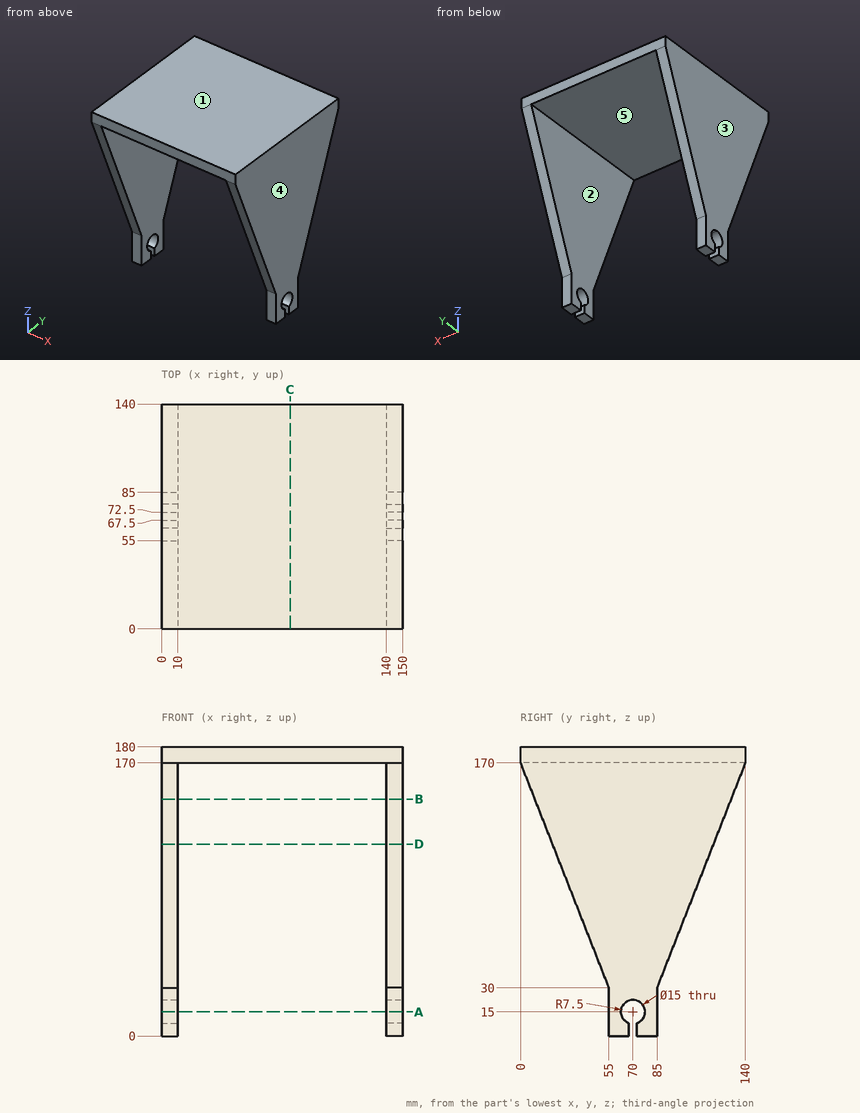
Source: three-view drawing plus pictorial views. Frame: mm from the lowest corner of the part. A direction names the side the tool comes from. Round coordinates to 2 decimals unless told otherwise and drop trailing zeros. Loops run counter-clockwise (first coordinate to the right, second up) from the corner with the lowest first, then second, coordinate; pieces in that order, holes last. Notation, with made-up numbers: (-28.5, 75.5) - (9.5, 75.5) arc R24 cw to (9.5, 87.5) - close; hole circle Ø7 at (63, 49.5). An arc over 180 degrees is marked (long way). Write each question's results on one line, items separated by ' | '. Start each with the question number.
1) Cut plane C-C on x = 80. Return loops of the section in (y, z).
2) Cut plane A-A on z = 15. Return loops of the section in (x, y).
3) Mould query, pull axis X, two halves, no side actions, for the marked faces 1, 2 and 3. Classes: released by +X, released by -X, zero draft, split by the parting line, or undercut.
4) First-contact query: P1, Ø6.5, axis at x = 5, z = 4.5, coming from the +Y side; P2, Ø5, axis at x = 5, z = 10, coming from the -Y side; P3, Ø12, axis at x = 64, y = 67.5, coming from the -Z side. Flat tips, straight axial feed; report the tip coordinate or a pass-through.
5) Line query: probe 1 along X at (y, z) = (81.5, 82); probe 2 along Y at (x, z) = (144.25, 15); probe 3 along Z at (x, y) = (13.5, 42.5). Output: solid intervals per line, ascending. Write a range as [from, to].
6) Cut plane B-B on z = 147.5. Return loops of the section in (x, y), then the cut area to 3 significant figures.
7) Access query for the marked faces 4 and 5. Directions: +Z, -Z, +X, -X, +Y, -Y. A direction counts if a zero-diameter tool reaches every point of the face in a straight line with its end or side. Return the directions, or none.
8) Cut plane D-D on z = 119.5. Return loops of the section in (x, y), then the cut area to 3 significant figures.
Verdict:
1) outline: (0, 170) - (140, 170) - (140, 180) - (0, 180) - close
2) outline: (0, 55) - (10, 55) - (10, 62.5) - (0, 62.5) - close; (0, 77.5) - (10, 77.5) - (10, 85) - (0, 85) - close; (140, 55) - (150, 55) - (150, 62.5) - (140, 62.5) - close; (140, 77.5) - (150, 77.5) - (150, 85) - (140, 85) - close
3) face 1: zero draft | face 2: undercut | face 3: released by -X
4) P1: stops at y = 85 | P2: stops at y = 55 | P3: stops at z = 170
5) probe 1: x = [0, 10], [140, 150] | probe 2: y = [55, 62.5], [77.5, 85] | probe 3: z = [170, 180]
6) outline: (0, 8.84) - (10, 8.84) - (10, 131.16) - (0, 131.16) - close; (140, 8.84) - (150, 8.84) - (150, 131.16) - (140, 131.16) - close | area: 2,450 mm2
7) face 4: +Z, -Z, +X, +Y, -Y | face 5: -Z, +Y, -Y
8) outline: (0, 19.84) - (10, 19.84) - (10, 120.16) - (0, 120.16) - close; (140, 19.84) - (150, 19.84) - (150, 120.16) - (140, 120.16) - close | area: 2,010 mm2
